Read the model definition and answer for the solid it produces. Units are mm, in the model's axes. A direction names the side the tool comes from. Give positions to 0.01 mm unless a question says otherwise; leave off trailing zeros. Order: outer loops, then holes, each group sorted by start corner. A loop starts at its lowest first (then second) coordinate and runs counter-clockwise, first axis right, second up. Notation, with made-up numbers: M -17,71.5 L 36,71.5 A33 ccw 36,108.5 Z; hole C 60,89.5 d10. An arc over 180 degrees is marked long. One line per item, written item: value.
Autodesk Inventor part; units mm, degrees
ref_plane "YZ Plane" through (0, 0, 0) normal (1, 0, 0) x (0, 1, 0)
ref_plane "XZ Plane" through (0, 0, 0) normal (0, 1, 0) x (-1, 0, 0)
ref_plane "XY Plane" through (0, 0, 0) normal (0, 0, 1) x (1, 0, 0)
sketch "Sketch1" plane through (0, 0, 0) normal (0, 0, 1) x (1, 0, 0)
  line L0 (-50.7247, 3.2468) -> (38.1753, 3.2468)
  line L1 (38.1753, 3.2468) -> (38.1753, -6.2782)
  line L2 (-50.7247, -6.2782) -> (-50.7247, 3.2468)
  line L3 (38.1753, -6.2782) -> (19.1253, -6.2782)
  line L4 (-50.7247, -6.2782) -> (-31.6747, -6.2782)
  line L5 (-31.6747, -6.2782) -> (-31.6747, -31.6782)
  line L6 (19.1253, -6.2782) -> (19.1253, -31.6782)
  line L7 (19.1253, -31.6782) -> (6.4253, -31.6782)
  line L8 (-31.6747, -31.6782) -> (-18.9747, -31.6782)
  line L9 (-18.9747, -31.6782) -> (-18.9747, -6.2782)
  line L10 (-18.9747, -6.2782) -> (6.4253, -6.2782)
  line L11 (6.4253, -6.2782) -> (6.4253, -31.6782)
  point P0 (0, 0)
  dimension "d0" = 88.9
  dimension "d1" = 9.525
  dimension "d2" = 19.05
  dimension "d3" = 19.05
  dimension "d4" = 25.4
  dimension "d5" = 12.7
  dimension "d6" = 12.7
extrude "Extrusion1" add sketch "Sketch1" against normal blind 50.8
sketch "Sketch2" plane through (-50.7247, 3.2468, 0) normal (0, 1, 0) x (1, 0, 0)
  line L0 (88.9, 50.8) -> (0, 50.8)
  line L1 (0, 0) -> (88.9, 0)
  line L2 (88.9, 0) -> (88.9, 50.8)
  line L3 (44.45, 0) -> (44.45, 50.8)
  point P0 (50.7247, 0)
  point P1 (82.55, 12.7)
  point P2 (82.55, 38.1)
  point P3 (6.35, 38.1)
  point P4 (6.35, 12.7)
  dimension "d9" = 44.45
  dimension "d10" = 38.1
  dimension "d11" = 38.1
  dimension "d12" = 38.1
  dimension "d13" = 38.1
  dimension "d14" = 25.4
  dimension "d15" = 25.4
  dimension "d16" = 12.7
  dimension "d17" = 12.7
hole "Hole1" at (31.8253, 3.2468, -12.7) at (31.8253, 3.2468, -38.1) at (-44.3747, 3.2468, -38.1) at (-44.3747, 3.2468, -12.7) direction (0, -1, 0) diameter 6.35 depth 25.4 tip angle 118
properties part number "8020_sliders"
1) Find section D-D, the plane y = 0. Write down the section's boundary in (x, z) (3 decimals).
Reported:
outline: M -50.725,-50.8 L 38.175,-50.8 L 38.175,0 L -50.725,0 Z; hole C -44.375,-38.1 d6.35; hole C -44.375,-12.7 d6.35; hole C 31.825,-38.1 d6.35; hole C 31.825,-12.7 d6.35
2) Find section B-B, the plane y = -17. Write down the section's boundary in (x, z), plus the area to 3 significant figures.
Reported:
outline: M -31.67,-50.8 L -18.97,-50.8 L -18.97,0 L -31.67,0 Z; M 6.43,-50.8 L 19.13,-50.8 L 19.13,0 L 6.43,0 Z
area: 1,290 mm^2
3) Consider probe 1 along X at (y, z) = (-2.5, -12.7); probe 2 along X at (y, z) = (-19, -36); probe 3 along Y at (x, z) = (34, -17.5). Determine where each line is inside the solid, lowest interval first.
Reported:
probe 1: x = -50.72 to -47.55, -41.2 to 28.65, 35 to 38.18
probe 2: x = -31.67 to -18.97, 6.43 to 19.13
probe 3: y = -6.28 to 3.25
4) Each of these flat-tipped pins is pushed along its axis until it touches: pin 1 Ø9.5 at (x, z) = (29, -37) entering from -Y; pin 2 Ø1.5 at (x, y) = (-24, -24) entering from +Z; pin 3 Ø4 at (y, z) = (-18, -5.5) entering from -X; pin 4 Ø4 at (x, z) = (31.83, -12.7) entering from +Y. Where does it stop, or does it pass through?
Reported:
pin 1: stops at y = -6.28
pin 2: stops at z = 0
pin 3: stops at x = -31.67
pin 4: passes through
5) Which of the six approach directions +Z, -Z, +X, -X, +Y, -Y give full straight-line access (tool end or side, diameter ignored) to faces 1 (the face through (-31.675, -19, -25)), 2 (the face through (-41.275, -1.582, -38.788)), 3 (the face through (-6, -6.278, -25)), 4 (the face through (19.125, -19, -25))?
Reported:
face 1: +Z, -Z, -X, -Y
face 2: +Y, -Y
face 3: +Z, -Z, -Y
face 4: +Z, -Z, +X, -Y
6) Find section A-A, the plane z = -12.7. Write down the section's boundary in (x, y).
Reported:
outline: M -50.72,-6.28 L -47.55,-6.28 L -47.55,3.25 L -50.72,3.25 Z; M -41.2,-6.28 L -31.67,-6.28 L -31.67,-31.68 L -18.97,-31.68 L -18.97,-6.28 L 6.43,-6.28 L 6.43,-31.68 L 19.13,-31.68 L 19.13,-6.28 L 28.65,-6.28 L 28.65,3.25 L -41.2,3.25 Z; M 35,-6.28 L 38.18,-6.28 L 38.18,3.25 L 35,3.25 Z
7) Find section C-C, the plane z = -22. Write down the section's boundary in (x, y), plus the area to 3 significant figures.
Reported:
outline: M -50.72,-6.28 L -31.67,-6.28 L -31.67,-31.68 L -18.97,-31.68 L -18.97,-6.28 L 6.43,-6.28 L 6.43,-31.68 L 19.13,-31.68 L 19.13,-6.28 L 38.18,-6.28 L 38.18,3.25 L -50.72,3.25 Z
area: 1,490 mm^2
8) Determine the mould class of faces 5 (the face through (38.175, -1, -25)), 6 (the face through (-7, 3.247, -25)), 7 (the face through (-50.725, -2, -25)), 8 (the face through (6.425, -19, -25)) for opening direction X: +X half, -X half, draft (parallel to the pull), parting line (faces both ways), or undercut.
Reported:
face 5: +X half
face 6: draft
face 7: -X half
face 8: undercut
